Input: part model. Units: mm. Frame: model coordinates. A direction names the side the tool comes from. Give positions to 0.01 mm unless a question says otherwise; leave off trailing zeros. Loops run counter-clockwise (first coordinate to the right, second up) from the corner with the lowest first, then second, coordinate; pieces in that order, holes last. Notation, with made-up numbers: M 62,53 L 101,53 A25 ccw 101,87 Z; hole C -11.5,84 d3. An arc over 180 degrees is marked long. Use CSV: the item, a comma, the result in double quotes. Start each with the question number.
Q1. Pull-direction query (Z, two-part tool) for faces 4 (the flat face through (78, -40, 0)), 5 (the cylindrical face through (116, -33, 0)); classes: released by +Z, released by -Z, zero draft, split by the parting line, or undercut.
Q2. Reachability of faces 1 (the flat face through (154, -25, 5)), 2 (the flat face through (85, -18, -3)), 3 (the flat face through (155, -33, 4)) from +Z, -Z, +X, -X, +Y, -Y: full face, straight path, thin tool, end or side. Return the list, or none.
Q3. Section C-C, the plane y = 30. Output: boundary loops of the cut face in (x, z).
Q4. Material intervals for line 1 along Y through (x, z) = (96, 0); line 2 along Y through (x, z) = (0, -3); line 3 along Y through (x, z) = (0, 1.5), sorted ascending.
Q5. Section D-D, the plane x = -12.5. Output: boundary loops of the cut face in (y, z), plus the area to 3 significant figures.
Q6. Section B-B, the plane x = 71. Output: boundary loops of the cut face in (y, z).
Q7. Pin query (flat end, axial travel): pin 1 (1.5 mm diameter, centred on y = -30.5, z = -3.5, fed in from -X); pin 2 (5 mm diameter, centred on y = -4, z = 5.5, fed in from -X); pin 3 (4.5 mm diameter, centred on y = -2, z = 3.5, fed in from +X). Return the tip coordinate at first contact, or that it passes through.
Q8. Section A-A, the plane x = 142. Output: boundary loops of the cut face in (y, z), plus the area to 3 significant figures.
from build123d import *

# Parameters (mm, degrees)
ESTRUSIONE1_DEPTH        = 7.5
SCHIZZO2_R               = 4
TAGLIO_ESTRUSIONE1_DEPTH = 15
SCHIZZO4_R               = 6.75
TAGLIO_ESTRUSIONE3_DEPTH = 8.5
SCHIZZO11_W              = 15
SCHIZZO11_H              = 15
ESTRUSIONE3_DEPTH        = 100
RACCORDO2_R              = 5
SCHIZZO13_R              = 4
TAGLIO_ESTRUSIONE4_DEPTH = 151.602954818
SCHIZZO14_R              = 7
TAGLIO_ESTRUSIONE5_DEPTH = 132.458168383
TAGLIO_ESTRUSIONE6_DEPTH = 100


with BuildPart() as part:
    # Schizzo1 → Estrusione1 (new, symmetric)
    with BuildSketch(Plane.XY):
        with BuildLine():
            Line((0, 40), (105, 40))
            Line((105, 40), (105, -40))
            Line((105, -40), (0, -40))
            ThreePointArc((0, -40), (-40, 0), (0, 40))
        make_face()
    extrude(amount=ESTRUSIONE1_DEPTH, both=True)

    # Schizzo2 → Taglio-Estrusione1 (cut)
    with BuildSketch(Plane.XY.offset(7.5)):
        Circle(SCHIZZO2_R)
    extrude(amount=-TAGLIO_ESTRUSIONE1_DEPTH, mode=Mode.SUBTRACT)

    # Schizzo4 → Taglio-Estrusione3 (cut)
    with BuildSketch(Plane.XY.offset(7.5)):
        Circle(SCHIZZO4_R)
    extrude(amount=-TAGLIO_ESTRUSIONE3_DEPTH, mode=Mode.SUBTRACT)

    # Schizzo11 → Estrusione3 (add)
    with BuildSketch(Plane(origin=(105, 0, 0), x_dir=(0, 0, -1), z_dir=(1, 0, 0))):
        with Locations((0, -32.5)):
            Rectangle(SCHIZZO11_W, SCHIZZO11_H)
    extrude(amount=ESTRUSIONE3_DEPTH)

    # Raccordo2
    raccordo2_edges = [part.edges().sort_by_distance(p)[0] for p in [
        (105, -25, 0),
        (205, -25, 0),
    ]]
    fillet(raccordo2_edges, radius=RACCORDO2_R)

    # Schizzo13 → Taglio-Estrusione4 (cut, through all)
    with BuildSketch(Plane(origin=(105, 0, 0), x_dir=(0, 0, -1), z_dir=(1, 0, 0))):
        with Locations((0, -15)):
            Circle(SCHIZZO13_R)
        with Locations((0, 30)):
            Circle(SCHIZZO13_R)
    extrude(amount=-TAGLIO_ESTRUSIONE4_DEPTH, mode=Mode.SUBTRACT)

    # Schizzo14 → Taglio-Estrusione5 (cut, through all)
    with BuildSketch(Plane(origin=(85, 0, 0), x_dir=(0, 0, -1), z_dir=(1, 0, 0))):
        with Locations((0, 30)):
            Circle(SCHIZZO14_R)
        with Locations((0, -15)):
            Circle(SCHIZZO14_R)
    extrude(amount=-TAGLIO_ESTRUSIONE5_DEPTH, mode=Mode.SUBTRACT)

    # Schizzo15 → Taglio-Estrusione6 (cut)
    with BuildSketch(Plane.XZ.offset(40)):
        with BuildLine():
            Line((120, 4), (190, 4))
            ThreePointArc((190, 4), (194, 0), (190, -4))
            Line((190, -4), (120, -4))
            ThreePointArc((120, -4), (116, 0), (120, 4))
        make_face()
    extrude(amount=-TAGLIO_ESTRUSIONE6_DEPTH, mode=Mode.SUBTRACT)


solid = part.part
A:
1,face 4,"zero draft"
1,face 5,"undercut"
2,face 1,"+Z, -Z, +X, +Y"
2,face 2,"-X"
2,face 3,"+Y, -Y"
3,outline,"M -26.46,-7.5 L 105,-7.5 L 105,-4 L 85,-4 L 85,-7 L -26.46,-7 Z; M -26.46,7 L 85,7 L 85,4 L 105,4 L 105,7.5 L -26.46,7.5 Z"
4,line 1,"-40 to -19, -11 to 26, 34 to 40"
4,line 2,"-40 to -21.32, -8.68 to -4, 4 to 23.68, 36.32 to 40"
4,line 3,"-40 to -21.84, -8.16 to -6.75, 6.75 to 23.16, 36.84 to 40"
5,outline,"M -38,-7.5 L 38,-7.5 L 38,7.5 L -38,7.5 Z; hole C -15,0 d14; hole C 30,0 d14"
5,area,"832 mm^2"
6,outline,"M -40,-7.5 L 40,-7.5 L 40,7.5 L -40,7.5 Z; hole C -15,0 d14; hole C 30,0 d14"
7,pin 1,"x = -26.74"
7,pin 2,"x = -39.97"
7,pin 3,"x = 105"
8,outline,"M -40,-7.5 L -25,-7.5 L -25,-4 L -40,-4 Z; M -40,4 L -25,4 L -25,7.5 L -40,7.5 Z"
8,area,"105 mm^2"
